```python
from build123d import *

# Parameters (mm, degrees)
CROQUIS2_R              = 4.5
SALIENTE_EXTRUIR1_DEPTH = 3
CROQUIS3_R              = 1.25
SALIENTE_EXTRUIR2_DEPTH = 15
REDONDEO1_R             = 1.5


with BuildPart() as part:
    # Croquis2 → Saliente-Extruir1 (new body)
    with BuildSketch(Plane.XY):
        Circle(CROQUIS2_R)
        with BuildLine():
            ThreePointArc((2.471875, 0.373943825), (2.165063509, 1.25), (1.559782352, 1.953734632))
            ThreePointArc((1.559782352, 1.953734632), (1.0625, 1.840303983), (0.912092648, 2.327678458))
            ThreePointArc((0.912092648, 2.327678458), (0, 2.5), (-0.912092648, 2.327678458))
            ThreePointArc((-0.912092648, 2.327678458), (-1.0625, 1.840303983), (-1.559782352, 1.953734632))
            ThreePointArc((-1.559782352, 1.953734632), (-2.165063509, 1.25), (-2.471875, 0.373943825))
            ThreePointArc((-2.471875, 0.373943825), (-2.125, 0), (-2.471875, -0.373943825))
            ThreePointArc((-2.471875, -0.373943825), (-2.165063509, -1.25), (-1.559782352, -1.953734632))
            ThreePointArc((-1.559782352, -1.953734632), (-1.0625, -1.840303983), (-0.912092648, -2.327678458))
            ThreePointArc((-0.912092648, -2.327678458), (0, -2.5), (0.912092648, -2.327678458))
            ThreePointArc((0.912092648, -2.327678458), (1.0625, -1.840303983), (1.559782352, -1.953734632))
            ThreePointArc((1.559782352, -1.953734632), (2.165063509, -1.25), (2.471875, -0.373943825))
            ThreePointArc((2.471875, -0.373943825), (2.125, 0), (2.471875, 0.373943825))
        make_face(mode=Mode.SUBTRACT)
    extrude(amount=SALIENTE_EXTRUIR1_DEPTH)

    # Croquis3 → Saliente-Extruir2 (add)
    with BuildSketch(Plane(origin=(0, 0, 0), x_dir=(-1, 0, 0), z_dir=(0, 0, -1))):
        with BuildLine():
            Line((1.25, 10.825317547), (1.25, 14.25))
            ThreePointArc((1.25, 14.25), (0, 15.5), (-1.25, 14.25))
            Line((-1.25, 14.25), (-1.25, 10.825317547))
            ThreePointArc((-1.25, 10.825317547), (-1.919872981, 8.325317547), (-3.75, 6.495190528))
            ThreePointArc((-3.75, 6.495190528), (-5.303300859, 5.303300859), (-6.495190528, 3.75))
            ThreePointArc((-6.495190528, 3.75), (-8.325317547, 1.919872981), (-10.825317547, 1.25))
            Line((-10.825317547, 1.25), (-14.25, 1.25))
            ThreePointArc((-14.25, 1.25), (-15.5, 0), (-14.25, -1.25))
            Line((-14.25, -1.25), (-10.825317547, -1.25))
            ThreePointArc((-10.825317547, -1.25), (-8.325317547, -1.919872981), (-6.495190528, -3.75))
            ThreePointArc((-6.495190528, -3.75), (-5.303300859, -5.303300859), (-3.75, -6.495190528))
            ThreePointArc((-3.75, -6.495190528), (-1.919872981, -8.325317547), (-1.25, -10.825317547))
            Line((-1.25, -10.825317547), (-1.25, -14.25))
            ThreePointArc((-1.25, -14.25), (0, -15.5), (1.25, -14.25))
            Line((1.25, -14.25), (1.25, -10.825317547))
            ThreePointArc((1.25, -10.825317547), (1.919872981, -8.325317547), (3.75, -6.495190528))
            ThreePointArc((3.75, -6.495190528), (5.303300859, -5.303300859), (6.495190528, -3.75))
            ThreePointArc((6.495190528, -3.75), (8.325317547, -1.919872981), (10.825317547, -1.25))
            Line((10.825317547, -1.25), (14.25, -1.25))
            ThreePointArc((14.25, -1.25), (15.5, 0), (14.25, 1.25))
            Line((14.25, 1.25), (10.825317547, 1.25))
            ThreePointArc((10.825317547, 1.25), (8.325317547, 1.919872981), (6.495190528, 3.75))
            ThreePointArc((6.495190528, 3.75), (5.303300859, 5.303300859), (3.75, 6.495190528))
            ThreePointArc((3.75, 6.495190528), (1.919872981, 8.325317547), (1.25, 10.825317547))
        make_face()
        Circle(CROQUIS3_R, mode=Mode.SUBTRACT)
    extrude(amount=SALIENTE_EXTRUIR2_DEPTH)

    # Redondeo1
    redondeo1_edges = [part.edges().sort_by_distance(p)[0] for p in [
        (-4.5, 0, 0),
    ]]
    fillet(redondeo1_edges, radius=REDONDEO1_R)


solid = part.part
```
Here's how the part is built. I have some questions about the finished solid (model axes, mm). A direction names the side the tool comes from. Give positions to 0.01 mm unless a question says otherwise; leave off trailing zeros. Order: outer loops, then holes, each group sorted by start corner. A loop starts at its lowest first (then second) coordinate and runs counter-clockwise, first axis right, second up. Notation, with made-up numbers: M -31.5,29 L -22.5,29 A23 cw -22.5,50 Z; hole C 3.25,3.5 d9. An arc over 180 degrees is marked long. Use a Markdown table: item, result. Add a question column.
1. If we mould it in two halves opening along Y, with no side actions, what happens to faces 5 (the cylindrical face through (0, -2.5, 1.5)), 6 (the cylindrical face through (5.323, -5.284, -7.395)), 7 (the cylindrical face through (0, 2.5, 1.5)), 8 (the flat face through (-1.25, -13, -7))? For each: +Y half, -Y half, draft (parallel to the pull), parting line (faces both ways), or undercut.
2. Suppose I cut it at D-D (y = 9). List the corners of the cut face in (x, z) for me.
3. Suppose I cut it at C-C (y = 13.5). List the corners of the cut face in (x, z) for me, and give its area (3 significant figures).
4. For pin 1 Ø2.5 at (x, z) = (-13, -4) entering from -Y; pin 2 Ø2.5 at (y, z) = (-13.5, -9) entering from -X; pin 3 Ø2.5 at (x, z) = (12.5, -9) entering from +Y; pin 4 Ø10 at (x, y) = (10.5, 8) entering from -Z, each with a flat end and sliding along its axis, tell me the tip position at first contact or that it passes through.
5. Suppose I cut it at B-B (z = -0.5). List the corners of the cut face in (x, y) for me, and give its area (3 significant figures).
6. I need wall thicknesses on probe 1 along Y at (x, z) = (0, -8.25); probe 2 along Z at (x, y) = (-0.5, -13); probe 3 along Y at (x, z) = (6.5, -7.25). Which ranges of each line are inside material? Lowest first, please. Write a range as from..to.
7. Suppose I cut it at A-A (x = 0). List the corners of the cut face in (y, z) for me, and give its area (3 significant figures).
8. On a 3-axis mill with a long thin cutter (end or side, diameter ignored), from which of +Z, -Z, +X, -X, +Y, -Y can I reach the whole of each face in a straight line? I mean faces 1 (the flat face through (-13, -1.25, -7)), 2 (the flat face through (-1, 1, 0)), 3 (the flat face through (13, -1.25, -7)), 4 (the flat face through (13, 1.25, -7)). Say none if no direction works.
Results list:
| question | item | result |
|---|---|---|
| 1 | face 5 | undercut |
| 1 | face 6 | -Y half |
| 1 | face 7 | undercut |
| 1 | face 8 | draft |
| 2 | outline | M -1.6,-15 L 1.6,-15 L 1.6,0 L -1.6,0 Z |
| 3 | outline | M -1.25,-15 L 1.25,-15 L 1.25,0 L -1.25,0 Z |
| 3 | area | 37.5 mm² |
| 4 | pin 1 | stops at y = -1.25 |
| 4 | pin 2 | stops at x = -1.25 |
| 4 | pin 3 | stops at y = 1.25 |
| 4 | pin 4 | passes through |
| 5 | outline | M -14.25,-1.25 L -10.83,-1.25 A5 cw -6.5,-3.75 A7.5 ccw -3.75,-6.5 A5 cw -1.25,-10.83 L -1.25,-14.25 A1.25 ccw 1.25,-14.25 L 1.25,-10.83 A5 cw 3.75,-6.5 A7.5 ccw 6.5,-3.75 A5 cw 10.83,-1.25 L 14.25,-1.25 A1.25 ccw 14.25,1.25 L 10.83,1.25 A5 cw 6.5,3.75 A7.5 ccw 3.75,6.5 A5 cw 1.25,10.83 L 1.25,14.25 A1.25 ccw -1.25,14.25 L -1.25,10.83 A5 cw -3.75,6.5 A7.5 ccw -6.5,3.75 A5 cw -10.83,1.25 L -14.25,1.25 A1.25 ccw Z; hole C 0,0 d2.5 |
| 5 | area | 264 mm² |
| 6 | probe 1 | y = -15.5..-1.25, 1.25..15.5 |
| 6 | probe 2 | z = -15..0 |
| 6 | probe 3 | y = -3.74..3.74 |
| 7 | outline | M -15.5,-15 L -1.25,-15 L -1.25,0 L -2.5,0 L -2.5,3 L -4.5,3 L -4.5,1.5 A1.5 cw -6,0 L -15.5,0 Z; M 1.25,-15 L 15.5,-15 L 15.5,0 L 6,0 A1.5 cw 4.5,1.5 L 4.5,3 L 2.5,3 L 2.5,0 L 1.25,0 Z |
| 7 | area | 440 mm² |
| 8 | face 1 | +Z, -Z, -X, -Y |
| 8 | face 2 | +Z |
| 8 | face 3 | +Z, -Z, +X, -Y |
| 8 | face 4 | +Z, -Z, +X, +Y |
